from build123d import *

# Parameters (mm, degrees)
F1_DEPTH       = 25
F2_D           = 5.5
F2_CSINK_D     = 11.2
F2_CSINK_ANGLE = 90


with BuildPart() as f1:
    # F0 (on Top) → F1 (new body)
    with BuildSketch(Plane.XY):
        Polygon((1.8908311613, -27.8043653816), (52.2800497711, -27.8043653816), (52.2800497711, 27.8043653816), (-16.5963244791, -8.826507852), align=None)
        Polygon((-52.2800497711, -27.8043653816), (1.8908311613, -27.8043653816), (-16.5963244791, -8.826507852), align=None)
        Polygon((-52.2800497711, 27.8043653816), (-52.2800497711, -27.8043653816), (-16.5963244791, -8.826507852), align=None)
        Polygon((-16.5963244791, -8.826507852), (52.2800497711, 27.8043653816), (-52.2800497711, 27.8043653816), align=None)
    extrude(amount=F1_DEPTH)

    # F2 (through all)
    with Locations(Plane(origin=(0, 0, 0), x_dir=(1, 0, 0), z_dir=(0, 0, -1))):
        with Locations((27.2964816114, -14.5172269666), (-16.5963244791, 8.826507852)):
            CounterSinkHole(F2_D / 2, F2_CSINK_D / 2, counter_sink_angle=F2_CSINK_ANGLE)


solid = f1.part
Source: CAD feature listing. Evaluate the final solid. Frame: model axes, mm. Give positions to 0.01 mm unless a question says otherwise; leave off trailing zeros. Write item = value, one per line. Start each with the question number.
Q1. Material intervals for probe 1 along Y at (x, z) = (27.5, 4); probe 2 along X at (y, z) = (13, 13); probe 3 along X at (y, z) = (-11, 22.75), sorted ascending.
Q2. Pin query (flat end, axial travel): pin 1 Ø7 at (x, y) = (-16.6, -8.83) entering from -Z; pin 2 Ø10 at (x, y) = (33, 8) entering from -Z; pin 3 Ø3.5 at (x, y) = (27.3, 14.52) entering from -Z. Return the tip coordinate at first contact, or that it passes through.
Q3. Draft query along X for faces 1 (the cylindrical face through (-14.414, -7.153, 14.08)), 2 (the flat face through (-1, -27.804, 12)), 3 (the cylindrical face through (25.818, 12.198, 14.08)), 4 (the flat face through (-52.28, 0, 12)). Return one class per face: +X half, -X half, draft (parallel to the pull), parting line (faces both ways), or undercut.
Computed values:
q1.probe_1 = -27.8 to 11.77, 17.26 to 27.8
q1.probe_2 = -52.28 to 25, 29.59 to 52.28
q1.probe_3 = -52.28 to -18.28, -14.91 to 52.28
q2.pin_1 = 2.09
q2.pin_2 = 0
q2.pin_3 = through
q3.face_1 = undercut
q3.face_2 = draft
q3.face_3 = undercut
q3.face_4 = -X half
